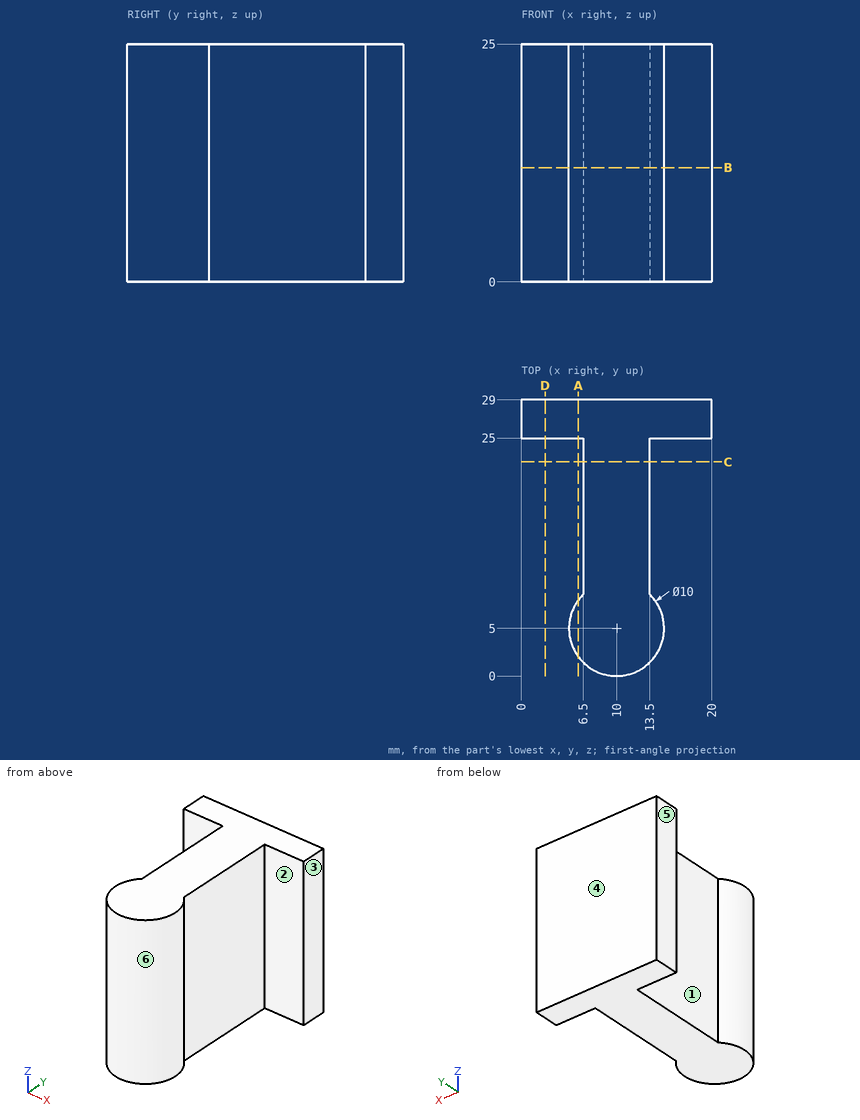
Here's the drawing with two shaded views (mm, measured from the low corner). I have some questions. A direction names the side the tool comes from. Coordinates: 2 decimals unless noted, no trailing zeros. Write each loop counter-clockwise with the first axis right and the second up, starting at its lowest first coordinate (ties: lowest second). Pieces come first, ordered by that corner, then holes. Notation, with made-up numbers: M 13,6.5 L 57,6.5 A21 ccw 57,42.5 Z; hole C 41.5,80 d10. An arc over 180 degrees is marked long. Answer as CSV lines item,"result".
Item 1: Please list where these lines run through material, in increasing order: line 1 along X through (y, z) = (15.75, 22.5); line 2 along Y through (x, z) = (2.25, 3.25); line 3 along Y through (x, z) = (5.5, 7.25).
Geometry results:
line 1,"x = 6.5 to 13.5"
line 2,"y = 25 to 29"
line 3,"y = 2.82 to 7.18, 25 to 29"
Item 2: Imagine slicing it at C-C on y = 22.5. List the corners of the cut face in (x, z) for me.
Geometry results:
outline,"M 6.5,0 L 13.5,0 L 13.5,25 L 6.5,25 Z"
Item 3: We'd pull the mould along Y, two halves only. Please class the marked faces 4, 5 and 6: +Y half, -Y half, draft (parallel to the pull), parting line (faces both ways), or undercut.
Geometry results:
face 4,"+Y half"
face 5,"draft"
face 6,"undercut"
Item 4: I'm going to push flat-ended pins straight in: P1, Ø1.5, axis at y = 16.5, z = 11, coming from the -X side; P2, Ø5, axis at x = 2.5, y = 13.5, coming from the -Z side; P3, Ø8, axis at y = 6, z = 10.5, coming from the -X side; P4, Ø6, axis at y = 14.5, z = 13, coming from the +X side. Where does each tip first touch, or does it pass through?
Geometry results:
P1,"stops at x = 6.5"
P2,"passes through"
P3,"stops at x = 5"
P4,"stops at x = 13.5"
Item 5: Imagine slicing it at A-A on x = 6. List the corners of the cut face in (y, z) for me.
Geometry results:
outline,"M 2,0 L 8,0 L 8,25 L 2,25 Z; M 25,0 L 29,0 L 29,25 L 25,25 Z"
Item 6: Imagine slicing it at B-B on z = 12. List the corners of the cut face in (x, y) for me.
Geometry results:
outline,"M 0,25 L 6.5,25 L 6.5,8.57 A5 ccw long 13.5,8.57 L 13.5,25 L 20,25 L 20,29 L 0,29 Z"
Item 7: On a 3-axis mill with a long thin cutter (end or side, diameter ignored), from which of +Z, -Z, +X, -X, +Y, -Y can I reach the whole of each face in a straight line? I mean the marked faces 1, 2 and 3. Say none if no direction works.
Geometry results:
face 1,"+Z, -Z, -X"
face 2,"+Z, -Z, +X"
face 3,"+Z, -Z, +X, +Y, -Y"
Item 8: Imagine slicing it at D-D on x = 2.5. List the corners of the cut face in (y, z) for me, plus the area to 3 significant figures.
Geometry results:
outline,"M 25,0 L 29,0 L 29,25 L 25,25 Z"
area,"100 mm2"
